Source: three-view drawing plus pictorial views. Frame: mm from the lowest corner of the part. Round coordinates to 2 decimals unless told otherwise and drop trailing zeros. Order: outer loops, then holes, each group sorted by start corner. A loop starts at its lowest first (then second) coordinate and runs counter-clockwise, first axis right, second up. Notation, with made-up numbers: M 19,21 L 66,21 A22 cw 66,59 Z; hole C -26.5,63.25 d5. An arc over 180 degrees is marked long. Return JSON: item names as keys, results as strings. Group by question number.
Q1. Cut plane C-C on y = 45. Output: boundary loops of the cut face in (x, z) (1 decimal), and give its area (3 significant figures).
Q2. Ray query, probe 1 along Y at (x, z) = (65.5, 43) (1 decimal); probe 2 along Z at (x, y) = (32.5, 29.5); probe 3 along X at (y, z) = (11, 57) (1 decimal). Return the intervals inside material, ascending.
Q3. Contact query for flat-ended pins moving along their axis: pin 1 (1.5 mm diameter, centred on y = 29.5, z = 10, fed in from +X) (1 decimal); pin 2 (1.5 mm diameter, centred on x = 10, z = 42.5, fed in from -Y) (1 decimal); pin 3 (2 mm diameter, centred on x = 31.5, z = 51.5, fed in from -Y) (1 decimal). Output: stop coordinate, or through.
Q4. Cut plane A-A on z = 35. Output: boundary loops of the cut face in (x, y) (1 decimal).
Q5. Mould query, pull axis X, two halves, no side actions, for the marked faces 1, 2 and 3. Classes: released by +X, released by -X, zero draft, split by the parting line, or undercut.
Q6. Cut plane B-B on x = 19. Output: boundary loops of the cut face in (y, z) (1 decimal).
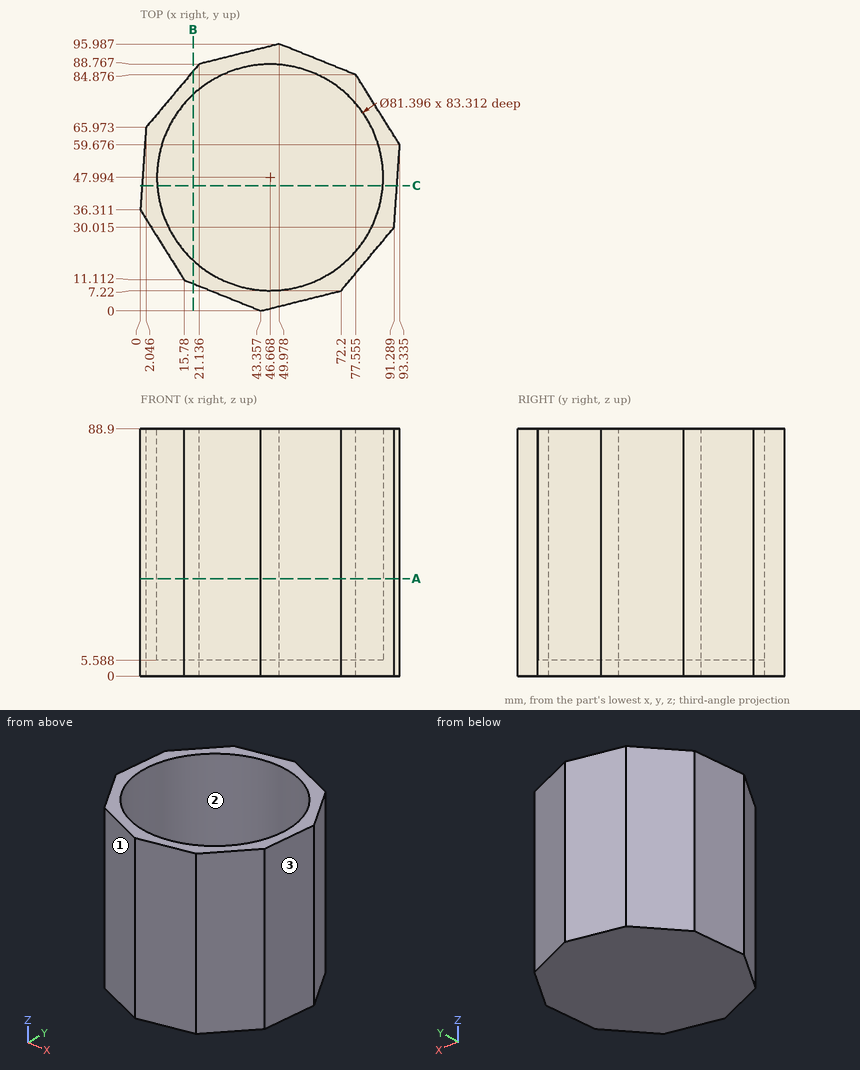
Result sheet:
{
 "1": {"outline": "M 0.6,0 L 92.3,0 L 92.3,88.9 L 87.3,88.9 L 87.3,5.6 L 6.1,5.6 L 6.1,88.9 L 0.6,88.9 Z", "area": "1,390 mm²"},
 "2": {"probe 1": "y = 5.5 to 11.9, 84.1 to 89.7", "probe 2": "z = 0 to 5.59", "probe 3": "x = 16.1 to 29.7, 63.6 to 75.4"},
 "3": {"pin 1": "stops at x = 91.3", "pin 2": "stops at y = 19.1", "pin 3": "stops at y = 4.4"},
 "4": {"outline": "M 0,36.3 L 15.8,11.1 L 43.4,0 L 72.2,7.2 L 91.3,30 L 93.3,59.7 L 77.6,84.9 L 50,96 L 21.1,88.8 L 2,66 Z; hole C 46.7,48 d81.4"},
 "5": {"face 1": "released by -X", "face 2": "undercut", "face 3": "released by +X"},
 "6": {"outline": "M 9.8,0 L 86.2,0 L 86.2,88.9 L 77.8,88.9 L 77.8,5.6 L 18.1,5.6 L 18.1,88.9 L 9.8,88.9 Z"}
}
